from build123d import *

# Parameters (mm, degrees)
SKETCH1_R                  = 6
SKETCH1_R_2                = 4
MAIN_DEPTH                 = 9.5
SKETCH2_W                  = 20
SKETCH2_H                  = 19
SKETCH2_R                  = 4
SKETCH2_R_2                = 1.35
BALLSUPPORTEXTRUSION_DEPTH = 5
SKETCH3_R                  = 5.15
BALLSUPPORTHOLE_DEPTH      = 4
FILLET2_R                  = 2


with BuildPart() as part:
    # Sketch1 → Main (new body, symmetric)
    with BuildSketch(Plane.XY):
        Circle(SKETCH1_R)
        Circle(SKETCH1_R_2, mode=Mode.SUBTRACT)
    extrude(amount=MAIN_DEPTH, both=True)

    # Sketch2 → BallSupportExtrusion (add)
    with BuildSketch(Plane(origin=(0, -9, 0), x_dir=(1, 0, 0), z_dir=(0, 1, 0))):
        with Locations((10, 0)):
            Rectangle(SKETCH2_W, SKETCH2_H)
        with Locations((13, 0)):
            Circle(SKETCH2_R, mode=Mode.SUBTRACT)
        with Locations((13, 7)):
            Circle(SKETCH2_R_2, mode=Mode.SUBTRACT)
        with Locations((13, -7)):
            Circle(SKETCH2_R_2, mode=Mode.SUBTRACT)
    extrude(amount=BALLSUPPORTEXTRUSION_DEPTH)

    # Sketch3 → BallSupportHole (cut)
    with BuildSketch(Plane(origin=(0, -4, 0), x_dir=(1, 0, 0), z_dir=(0, 1, 0))):
        with Locations((13, 0)):
            Circle(SKETCH3_R)
    extrude(amount=-BALLSUPPORTHOLE_DEPTH, mode=Mode.SUBTRACT)

    # Fillet2
    fillet2_edges = [part.edges().sort_by_distance(p)[0] for p in [
        (0, -6, 0),
        (4.472135955, -4, 0),
    ]]
    fillet(fillet2_edges, radius=FILLET2_R)


solid = part.part
Build history of the part. All positions in model axes, mm. A direction names the side the tool comes from. Coordinates: 2 decimals unless noted, no trailing zeros. Order: outer loops, then holes, each group sorted by start corner. A loop starts at its lowest first (then second) coordinate and runs counter-clockwise, first axis right, second up. Notation, with made-up numbers: M 29.25,80.25 L 54.25,80.25 A7 ccw 54.25,92.25 Z; hole C 84,30.5 d5. An arc over 180 degrees is marked long. One line per question, with ' | ' between items. Start each with the question number.
Q1. 3-axis set-ups, long thin cutter, end or side, ignore diameter. For faces 4 (the face through (7, -5, -9.5)), 5 (the face through (17.91, -5.97, -1.55)), 6 (the face through (18, -4, -2)), 7 (the face through (0, -8, 0)): which of +Z, -Z, +X, -X, +Y, -Y reach the whole face in a straight line?
Q2. Saw through at B-B (z = 7). List the corners of the cut face in (x, y).
Q3. Probe L1, parallel to X at y = -7.6, z = 7; L2, parallel to Y at x = 9.25, z = -2; L3, parallel to Y at x = 3.5, z = 6.5. List the from-to ranges inside material, lowest first. Write a range as from..to.
Q4. Flat gauge pins, fed straight in: pin 1 Ø1 at (y, z) = (-2, -6) entering from -X; pin 2 Ø5 at (y, z) = (-3.5, -5) entering from +X; pin 3 Ø3 at (x, z) = (13, 7) entering from +Y; pin 4 Ø1 at (x, z) = (7, 7.5) entering from +Y. Where does each tip first touch, or does it go through?
Q5. Saw through at D-D (x = -3.5). List the corners of the cut face in (y, z), then the cut area to 3 significant figures.
Q6. Two-plate mould, pull along Y, no slides. Class faces 1 (the face through (16, -8, 3)), 2 (the face through (-0.867, -3.905, -0.133)), 3 (the face through (12.005, -6.535, 6.088)): +Y half, -Y half, draft (parallel to the pull), parting line (faces both ways), or undercut.
Q7. Saw through at C-C (y = 1.5). List the corners of the cut face in (x, z), then the cut area to 3 significant figures.
Q8. Saw through at A-A (x = 13). List the corners of the cut face in (y, z), then the cut area to 3 significant figures.
Check values:
1) face 4: -Z, +X, -X, +Y, -Y | face 5: +Y | face 6: +Z, -Z, +X, +Y | face 7: +Z, -Z, -X, -Y
2) outline: M -1.5,-5.81 A2 cw 0,-7.75 L 0,-9 L 11.65,-9 L 11.65,-4 L 7.75,-4 A2 cw 5.81,-1.5 A6 ccw long Z; M 14.35,-9 L 20,-9 L 20,-4 L 14.35,-4 Z; hole C 0,0 d8
3) L1: x = -0.01..11.65, 14.35..20 | L2: y = -9..-8 | L3: y = -9..-1.94, 1.94..4.87
4) pin 1: stops at x = -5.81 | pin 2: stops at x = 20 | pin 3: stops at y = -4 | pin 4: stops at y = -3.56
5) outline: M -4.87,-9.5 L -1.94,-9.5 L -1.94,9.5 L -4.87,9.5 Z; M 1.94,-9.5 L 4.87,-9.5 L 4.87,9.5 L 1.94,9.5 Z | area: 112 mm2
6) face 1: +Y half | face 2: undercut | face 3: draft
7) outline: M -5.81,-9.5 L -3.71,-9.5 L -3.71,9.5 L -5.81,9.5 Z; M 3.71,-9.5 L 5.81,-9.5 L 5.81,9.5 L 3.71,9.5 Z | area: 79.9 mm2
8) outline: M -9,-9.5 L -4,-9.5 L -4,-8.35 L -9,-8.35 Z; M -9,-5.65 L -4,-5.65 L -4,-5.15 L -8,-5.15 L -8,-4 L -9,-4 Z; M -9,4 L -8,4 L -8,5.15 L -4,5.15 L -4,5.65 L -9,5.65 Z; M -9,8.35 L -4,8.35 L -4,9.5 L -9,9.5 Z | area: 18.8 mm2
